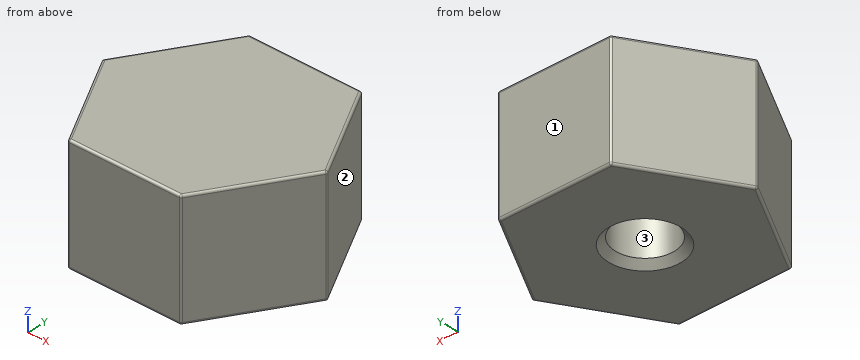
Autodesk Fusion 360 part; units mm, degrees
sketch "Sketch1" plane through (0, 0, 0) normal (0, 0, 1) x (1, 0, 0)
  line L0 (8, -8) -> (-8, -8)
  line L1 (-8, -8) -> (-8, 8)
  line L2 (-8, 8) -> (8, 8)
  line L3 (8, 8) -> (8, -8)
  line L4 (8, -8) -> (-8, 8) construction
  line L5 (-8, -8) -> (8, 8) construction
  circle A0 centre (0, 0) radius 2.575
  circle A1 centre (0, 0) radius 3.05
  line L6 (10, 0) -> (5, 8.6603)
  line L7 (5, 8.6603) -> (-5, 8.6603)
  line L8 (-5, 8.6603) -> (-10, 0)
  line L9 (-10, 0) -> (-5, -8.6603)
  line L10 (-5, -8.6603) -> (5, -8.6603)
  line L11 (5, -8.6603) -> (10, 0)
  dimension "d1" = 16
  dimension "d2" = 16
  dimension "d20" = 5.15
  dimension "d23" = 6.1
  dimension "d28" = 10
extrude "Extrude1" add sketch "Sketch1" along normal blind 10 contours L0 L9 L10 L11 | L0 L1 L2 L3 L6 L8 L9 L11 | L3 L6 L11 | L1 L8 L9 | L2 L6 L7 L8 | A0 | A1
fillet "Fillet1" radius 0.2 7 faces at (3.3333, 0, 10) (-1.6667, -8.6603, 3.3333) (8.3333, -2.8868, 6.6667) (-8.3333, -2.8868, 3.3333) (-6.6667, 5.7735, 3.3333) (1.6667, 8.6603, 3.3333) (8.3333, 2.8868, 3.3333)
extrude "Extrude5" cut sketch "Sketch1" along normal blind 8 contours A0
chamfer "Chamfer3" distance 0.6 angle 45 1 edges at (-2.4007, -0.9312, 0)
The listing builds one solid part. Answer for the finished solid, in the listing's coordinates (mm). Face numbers are marked on the shaded views. Give positions to 0.01 mm unless a question says otherwise; leave off trailing zeros. Write each loop counter-clockwise with the first axis right and the second up, starting at its lowest first coordinate (ties: lowest second). Pieces come first, ordered by that corner, then holes. Notation, with made-up numbers: (-29, -27) -> (24, -27) arc R26 cw to (24, -3) -> close; hole circle Ø9 at (11.5, 22). An arc over 180 degrees is marked (long way). Write item = value, one per line. Start each with the question number.
1) Each of these flat-tipped pins is pushed along its axis until it touches: pin 1 (1 mm diameter, centred on y = 2, z = 5, fed in from +X); pin 2 (4.5 mm diameter, centred on x = 0, y = 0, fed in from -Z). Where does it stop, or does it pass through?
2) The part is cut by section C-C, the plane z = 6. Determine the outline of the cut face in (x, y) (3 decimals).
3) Determine the mould class of the marked faces 1, 2 and 3 for opening direction X: +X half, -X half, draft (parallel to the pull), parting line (faces both ways), or undercut.
4) Straight lines are drawn through the part: line 1 along Y through (x, z) = (0, 3.25) (3 decimals); line 2 along X through (y, z) = (-0.5, 6.25); line 3 along X through (y, z) = (-7, 4.75). For each, find the intervals that lie inside material, in ascending order.
5) The part is cut by section A-A, the plane z = 9. Determine the outline of the cut face in (x, y), and give its area (3 significant figures).
6) The part is cut by section B-B, the plane x = 0. Determine the outline of the cut face in (y, z) (3 decimals), and give its area (3 significant figures).
Solutions:
q1.pin_1 = 9.13
q1.pin_2 = 8
q2.outline = (-9.942, -0.1) -> (-5.058, -8.56) arc R0.2 ccw to (-4.885, -8.66) -> (4.885, -8.66) arc R0.2 ccw to (5.058, -8.56) -> (9.942, -0.1) arc R0.2 ccw to (9.942, 0.1) -> (5.058, 8.56) arc R0.2 ccw to (4.885, 8.66) -> (-4.885, 8.66) arc R0.2 ccw to (-5.058, 8.56) -> (-9.942, 0.1) arc R0.2 ccw to start; hole circle Ø5.15 at (0, 0)
q3.face_1 = draft
q3.face_2 = +X half
q3.face_3 = undercut
q4.line_1 = -8.66 to -2.575, 2.575 to 8.66
q4.line_2 = -9.71 to -2.53, 2.53 to 9.71
q4.line_3 = -5.96 to 5.96
q5.outline = (-9.94, -0.1) -> (-5.06, -8.56) arc R0.2 ccw to (-4.88, -8.66) -> (4.88, -8.66) arc R0.2 ccw to (5.06, -8.56) -> (9.94, -0.1) arc R0.2 ccw to (9.94, 0.1) -> (5.06, 8.56) arc R0.2 ccw to (4.88, 8.66) -> (-4.88, 8.66) arc R0.2 ccw to (-5.06, 8.56) -> (-9.94, 0.1) arc R0.2 ccw to start
q5.area = 260 mm²
q6.outline = (-8.66, 0.2) arc R0.2 ccw to (-8.46, 0) -> (-3.175, 0) -> (-2.575, 0.6) -> (-2.575, 8) -> (2.575, 8) -> (2.575, 0.6) -> (3.175, 0) -> (8.46, 0) arc R0.2 ccw to (8.66, 0.2) -> (8.66, 9.8) arc R0.2 ccw to (8.46, 10) -> (-8.46, 10) arc R0.2 ccw to (-8.66, 9.8) -> close
q6.area = 132 mm²
